Print and shaded views of the part. All mm, measured from the part's lowest x, y and z. Coordinates: 2 decimals unless noted, no trailing zeros. Write each loop counter-clockwise with the first axis right and the second up, starting at its lowest first coordinate (ties: lowest second). Pieces come first, ordered by that corner, then holes. Notation, with made-up numbers: (77, 51) -> (105, 51) arc R22 ccw to (105, 76) -> close; hole circle Ø4 at (56, -19). An arc over 180 degrees is marked (long way). Write item = value, one per line.
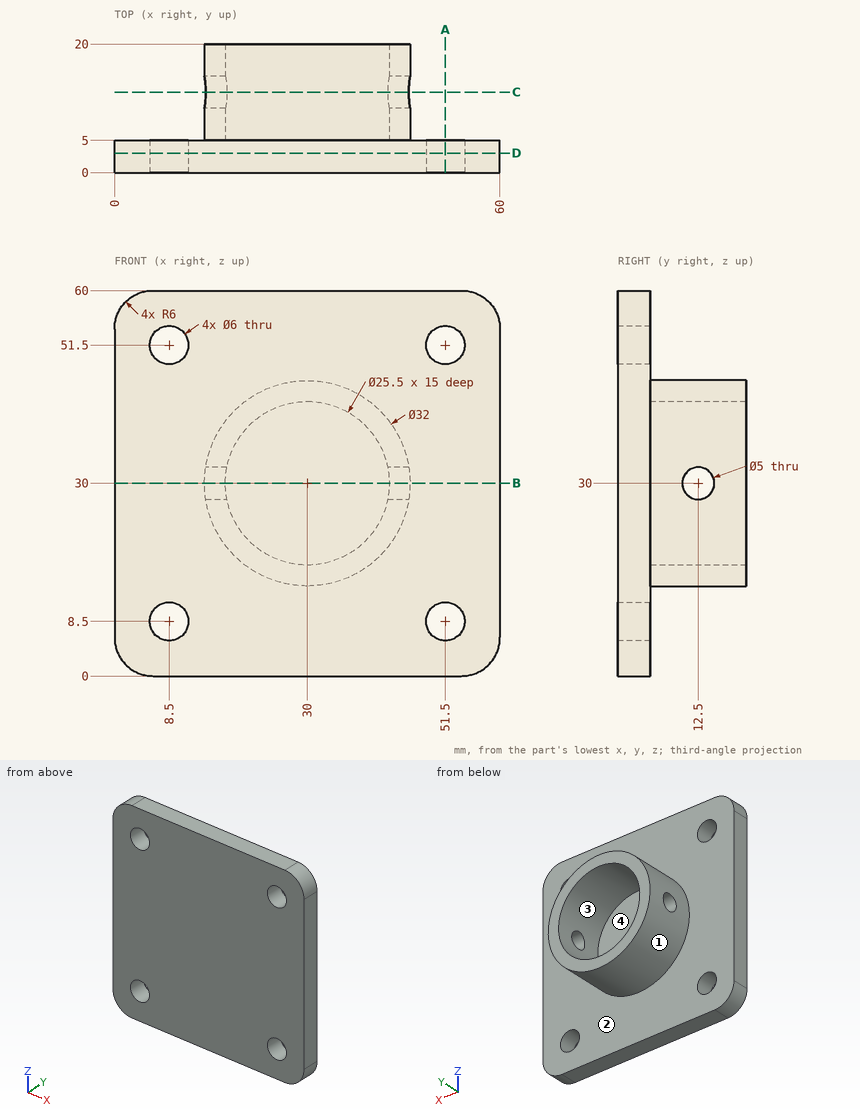
Q1. Probe line 1 (X direction, y = 1.65, z = 8.5); line 2 (Y direction, x = 53.5, z = 49); line 3 (Z direction, x = 15.35, y = 12.5). List the from-to ranges inside material, lowest first. Write a range as from..to.
Model answer:
line_1 = 0..5.5, 11.5..48.5, 54.5..60
line_2 = 0..5
line_3 = 23.57..27.5, 32.5..36.43
Q2. Saw through at C-C on y = 12.5. Give the cut face in (x, z), and give its area (3 significant figures).
Model answer:
outline = (14.2, 27.5) arc R16 ccw to (45.8, 27.5) -> (42.5, 27.5) arc R12.75 cw to (17.5, 27.5) -> close; (14.2, 32.5) -> (17.5, 32.5) arc R12.75 cw to (42.5, 32.5) -> (45.8, 32.5) arc R16 ccw to start
area = 261 mm²
Q3. Saw through at B-B on z = 30. Give the cut face in (x, y), and give its area (3 significant figures).
Model answer:
outline = (0, 0) -> (60, 0) -> (60, 5) -> (46, 5) -> (46, 10) -> (42.75, 10) -> (42.75, 5) -> (17.25, 5) -> (17.25, 10) -> (14, 10) -> (14, 5) -> (0, 5) -> close; (14, 15) -> (17.25, 15) -> (17.25, 20) -> (14, 20) -> close; (42.75, 15) -> (46, 15) -> (46, 20) -> (42.75, 20) -> close
area = 365 mm²
Q4. Mould opens along X. For the marked faces 1, 2, 3 and 4 say: released by +X, released by -X, zero draft, split by the parting line, or undercut.
Model answer:
face_1 = split by the parting line
face_2 = zero draft
face_3 = undercut
face_4 = undercut
Q5. Saw through at A-A on x = 51.5. Give the cut face in (y, z).
Model answer:
outline = (0, 0) -> (5, 0) -> (5, 5.5) -> (0, 5.5) -> close; (0, 11.5) -> (5, 11.5) -> (5, 48.5) -> (0, 48.5) -> close; (0, 54.5) -> (5, 54.5) -> (5, 60) -> (0, 60) -> close
Q6. Pin check, flat tips, straight feed: pin 1 (4 mm diameter, centred on x = 45, y = 11.5, fed in from +Z); pin 2 (2 mm diameter, centred on x = 18, y = 8.5, fed in from -Z); pin 3 (8 mm diameter, centred on x = 51.5, z = 8.5, fed in from +Y). Stop position of each tip, or through.
Model answer:
pin_1 = 39.33
pin_2 = 18.38
pin_3 = 5
Q7. Saw through at D-D on y = 3. Give the cut face in (x, z).
Model answer:
outline = (0, 6) arc R6 ccw to (6, 0) -> (54, 0) arc R6 ccw to (60, 6) -> (60, 54) arc R6 ccw to (54, 60) -> (6, 60) arc R6 ccw to (0, 54) -> close; hole circle Ø6 at (8.5, 8.5); hole circle Ø6 at (8.5, 51.5); hole circle Ø6 at (51.5, 8.5); hole circle Ø6 at (51.5, 51.5)
